Verification items for this drawing (mm, ordinates from the low corner). Round coordinates to 2 decimals unless told otherwise and drop trailing zeros. Loops run counter-clockwise (first coordinate to the right, second up) from the corner with the lowest first, then second, coordinate; pieces in that order, holes last. Notation, with made-up numbers: M -16,52.5 L 42,52.5 A20 ccw 42,89.5 Z; hole C -21.5,19 d5. An arc over 180 degrees is marked long. Write item = value, one per line. Start each with the question number.
(1) Cross-section at B-B on x = 8.5. Record the boundary of the cut face in (y, z) (1 decimal).
(2) Cross-section at C-C on y = 1.05. State how many separate pieces and enclosed holes the cut face has.
(3) Go/stop test with flat-tipped pins: P1, Ø1, axis at x = 13.5, y = 1.5, coming from the -Z side (1 decimal); P2, Ø5.5, axis at x = 7.94, z = 33.34, coming from the +Y side. Record where each tip stops, or that it passes through.
(4) Cross-section at A-A on z = 9. Record the boundary of the cut face in (x, y) (1 decimal), plus the area to 3 significant figures.
(5) Cross-section at D-D on z = 32.5. Record the boundary of the cut face in (x, y) (1 decimal).
(6) Scan lines: L1, parallel to Z at x = 7.75, y = 1.6; L2, parallel to Z at x = 9.75, y = 1.6 (1 decimal); L3, parallel to X at y = 1.35, z = 56.5 (1 decimal). Record each from-to range of solid material in increasing order. Write a range as from..to.
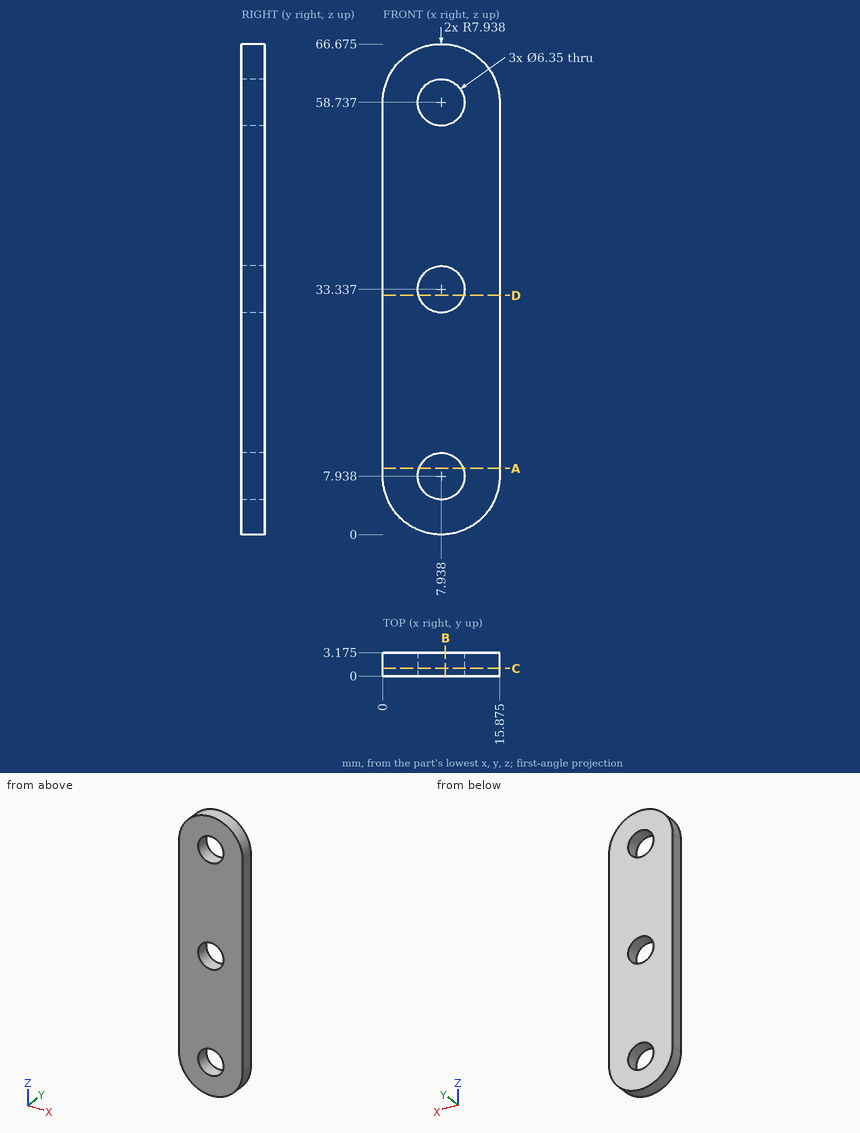
Result:
q1.outline = M 0,0 L 3.2,0 L 3.2,4.8 L 0,4.8 Z; M 0,11.1 L 3.2,11.1 L 3.2,30.2 L 0,30.2 Z; M 0,36.5 L 3.2,36.5 L 3.2,55.6 L 0,55.6 Z; M 0,61.9 L 3.2,61.9 L 3.2,66.7 L 0,66.7 Z
q2.separate_pieces = 1
q2.enclosed_holes = 3
q3.P1 = 1.8
q3.P2 = through
q4.outline = M 0,0 L 4.9,0 L 4.9,3.2 L 0,3.2 Z; M 10.9,0 L 15.9,0 L 15.9,3.2 L 10.9,3.2 Z
q4.area = 31.4 mm^2
q5.outline = M 0,0 L 4.9,0 L 4.9,3.2 L 0,3.2 Z; M 11,0 L 15.9,0 L 15.9,3.2 L 11,3.2 Z
q6.L1 = 0..4.77, 11.11..30.17, 36.51..55.57, 61.91..66.67
q6.L2 = 0.2..5.3, 10.5..30.7, 35.9..56.1, 61.3..66.5
q6.L3 = 0..5.7, 10.2..15.9
